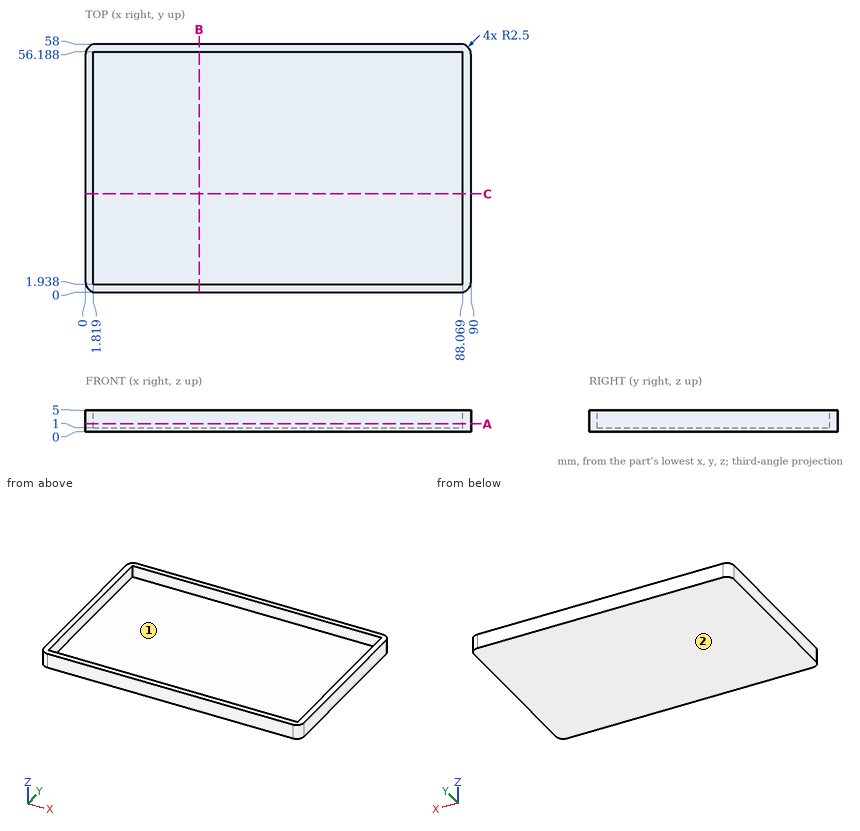
Geometry check sheet. Reference: drawing and pictorial views, mm from the part's lowest x, y, z. Coordinates: 2 decimals unless noted, no trailing zeros. Write each loop counter-clockwise with the first axis right and the second up, starting at its lowest first coordinate (ties: lowest second). Pieces come first, ordered by that corner, then holes. Notation, with made-up numbers: (23, 61.5) -> (76, 61.5) arc R14 cw to (76, 75.5) -> close; hole circle Ø7 at (8.5, 33). An arc over 180 degrees is marked (long way). Use a Markdown table: item, result.
1. Scan lines: line 1 along Y through (x, z) = (56, 4.75); line 2 along X through (y, z) = (45, 3.7); line 3 along Z through (x, y) = (34.5, 41). Record each from-to range of solid material in increasing order.
Reported:
| item | result |
|---|---|
| line 1 | y = 0 to 1.94, 56.19 to 58 |
| line 2 | x = 0 to 1.82, 88.07 to 90 |
| line 3 | z = 0 to 1 |
2. Release check for a two-part mould opening along X. For the marked faces 1 and 2 record: pulls with the +X half, pulls with the -X half, needs draft (parallel to the pull), parting line crosses it, or undercut.
Reported:
| item | result |
|---|---|
| face 1 | undercut |
| face 2 | needs draft |
3. Sectioned sample at B-B (x = 26.5). Enter the section's corners in (y, z).
Reported:
| item | result |
|---|---|
| outline | (0, 0) -> (58, 0) -> (58, 5) -> (56.19, 5) -> (56.19, 1) -> (1.94, 1) -> (1.94, 5) -> (0, 5) -> close |
4. Sectioned sample at A-A (z = 1.85). Enter the section's corners in (x, y).
Reported:
| item | result |
|---|---|
| outline | (0, 2.5) arc R2.5 ccw to (2.5, 0) -> (87.5, 0) arc R2.5 ccw to (90, 2.5) -> (90, 55.5) arc R2.5 ccw to (87.5, 58) -> (2.5, 58) arc R2.5 ccw to (0, 55.5) -> close; hole (1.82, 1.94) -> (88.07, 1.94) -> (88.07, 56.19) -> (1.82, 56.19) -> close |
5. Sectioned sample at C-C (y = 23). Enter the section's corners in (x, z), plus the area to 3 significant figures.
Reported:
| item | result |
|---|---|
| outline | (0, 0) -> (90, 0) -> (90, 5) -> (88.07, 5) -> (88.07, 1) -> (1.82, 1) -> (1.82, 5) -> (0, 5) -> close |
| area | 105 mm2 |
6. Go/stop test with a flat-tipped pin: pin 1 Ø10 at (x, y) = (61.5, 45) entering from +Z. Record where the tip stops, or that it passes through.
Reported:
| item | result |
|---|---|
| pin 1 | stops at z = 1 |
